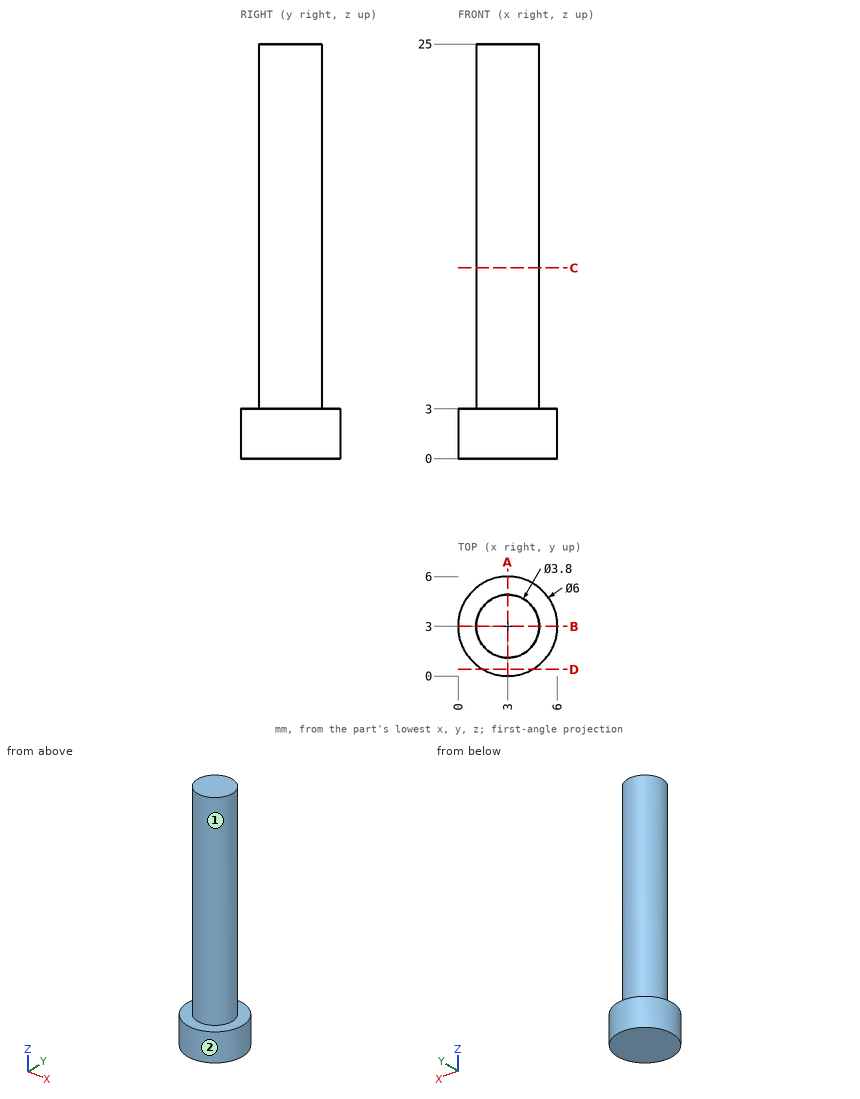
Answer from the drawing. Dimensions are ordinates in mm from the lowest x, y and z of the part. A direction names the side the tool comes from. Give positions to 0.01 mm unless a question says otherwise; leave off trailing zeros. Loops run counter-clockwise (first coordinate to the right, second up) from the corner with the lowest first, then second, coordinate; pieces in that order, holes last. Notation, with made-up numbers: (-35.75, -15.5) -> (-0.75, -15.5) arc R35 cw to (-0.75, 18.5) -> close; hole circle Ø8 at (-11, 16). An arc over 180 degrees is marked (long way). Use a Markdown table: item, result.
Q1. Section C-C, the plane z = 11.5 is taken. Determine the outline of the cut face in (x, y), then the cut area to 3 significant figures.
Solved:
| item | result |
|---|---|
| outline | circle Ø3.8 at (3, 3) |
| area | 11.3 mm^2 |
Q2. Section D-D, the plane y = 0.4 is taken. Determine the outline of the cut face in (x, z).
Solved:
| item | result |
|---|---|
| outline | (1.5, 0) -> (4.5, 0) -> (4.5, 3) -> (1.5, 3) -> close |
Q3. Each of these flat-tipped pins is pushed along its axis until it touches: pin 1 (1.5 mm diameter, centred on x = 5, y = 5, fed in from +Z); pin 2 (3 mm diameter, centred on y = 3.5, z = 11, fed in from -X); pin 3 (1 mm diameter, centred on y = 4, z = 22, fed in from +X). Where does it stop, or does it pass through?
Solved:
| item | result |
|---|---|
| pin 1 | stops at z = 3 |
| pin 2 | stops at x = 1.1 |
| pin 3 | stops at x = 4.83 |
Q4. Section A-A, the plane x = 3 is taken. Determine the outline of the cut face in (y, z).
Solved:
| item | result |
|---|---|
| outline | (0, 0) -> (6, 0) -> (6, 3) -> (4.9, 3) -> (4.9, 25) -> (1.1, 25) -> (1.1, 3) -> (0, 3) -> close |
Q5. Find the intervals of material crossed by line 1 along X through (y, z) = (3, 18.75); line 2 along Z through (x, y) = (0.85, 3.85), in increasing order.
Solved:
| item | result |
|---|---|
| line 1 | x = 1.1 to 4.9 |
| line 2 | z = 0 to 3 |
Q6. A tool of negligible diameter and unlimited length cuts with its end or side. For the marked faces 1 and 2, from which of +Z, -Z, +X, -X, +Y, -Y can it reach the whole face along a straight path? Write none if from no direction.
Solved:
| item | result |
|---|---|
| face 1 | +Z |
| face 2 | +Z, -Z |
